Build history of the part. All positions in model axes, mm. Face numbers are marked on the shaded views. Coordinates: 2 decimals unless noted, no trailing zeros. Order: outer loops, then holes, each group sorted by start corner. A loop starts at its lowest first (then second) coordinate and runs counter-clockwise, first axis right, second up. Notation, with made-up numbers: (12.5, 55) - (56.5, 55) arc R6 ccw to (56.5, 62) - close; hole circle Ø8 at (16.5, 17.25). An arc over 180 degrees is marked (long way). Write each question's results on one line, items separated by ' | '.
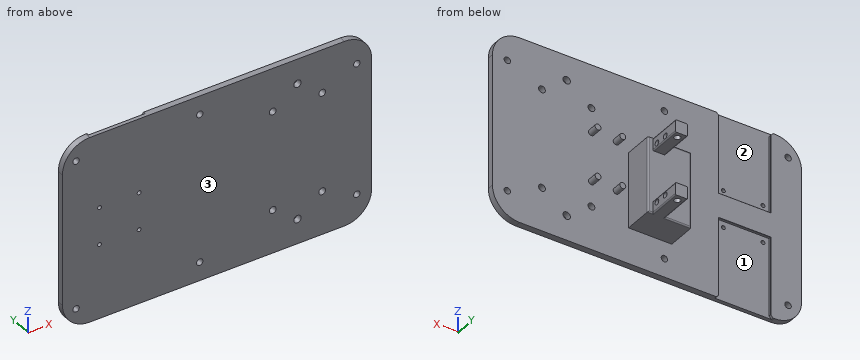
from build123d import *

# Parameters (mm, degrees)
SKETCH_1_R          = 2.6
SKETCH_1_R_2        = 3
SKETCH_1_R_3        = 2.75
EXTRUDE_1_DEPTH     = 5
SKETCH_2_W          = 42
SKETCH_2_H          = 65
CUT_EXTRUDE_1_DEPTH = 2
CHAMFER_1_SIZE      = 0.2
SKETCH_3_R          = 1.6
CUT_EXTRUDE_2_DEPTH = 3
CHAMFER_2_SIZE      = 2
SKETCH_4_R          = 2.4
EXTRUDE_2_DEPTH     = 8
SKETCH_5_W          = 35
SKETCH_5_H          = 61
EXTRUDE_3_DEPTH     = 23.5
SKETCH_7_W          = 35
SKETCH_7_H          = 10
EXTRUDE_4_DEPTH     = 30
SKETCH_8_W          = 4
SKETCH_8_H          = 10
SKETCH_8_W_2        = 21
CUT_EXTRUDE_3_DEPTH = 30
FILLET_1_R          = 1
SKETCH_9_R          = 2.2
CUT_EXTRUDE_4_DEPTH = 158.870991636
SKETCH_10_R         = 2.5
SKETCH_10_W         = 10
SKETCH_10_H         = 3
CUT_EXTRUDE_5_DEPTH = 165.764225486


with BuildPart() as part:
    # 草图1 → 凸台-拉伸1 (new body)
    with BuildSketch(Plane(origin=(0, 0, 0), x_dir=(1, 0, 0), z_dir=(0, 1, 0))):
        with BuildLine():
            Line((103, 75), (95, 75))
            Line((95, 75), (55, 75))
            Line((55, 75), (-103, 75))
            ThreePointArc((-103, 75), (-118.556349186, 68.556349186), (-125, 53))
            Line((-125, 53), (-125, -53))
            ThreePointArc((-125, -53), (-118.556349186, -68.556349186), (-103, -75))
            Line((-103, -75), (55, -75))
            Line((55, -75), (95, -75))
            Line((95, -75), (103, -75))
            ThreePointArc((103, -75), (118.556349186, -68.556349186), (125, -53))
            Line((125, -53), (125, 53))
            ThreePointArc((125, 53), (118.556349186, 68.556349186), (103, 75))
        make_face()
        with Locations(Location((-114, 60, 0), (0, 0, 270))):
            Circle(SKETCH_1_R, mode=Mode.SUBTRACT)
        with Locations(Location((-14, 60, 0), (0, 0, 270))):
            Circle(SKETCH_1_R, mode=Mode.SUBTRACT)
        with Locations(Location((113, 53, 0), (0, 0, 270))):
            Circle(SKETCH_1_R, mode=Mode.SUBTRACT)
        with Locations(Location((-114, -60, 0), (0, 0, 270))):
            Circle(SKETCH_1_R, mode=Mode.SUBTRACT)
        with Locations(Location((-14, -60, 0), (0, 0, 270))):
            Circle(SKETCH_1_R, mode=Mode.SUBTRACT)
        with Locations(Location((113, -53, 0), (0, 0, 270))):
            Circle(SKETCH_1_R, mode=Mode.SUBTRACT)
        with Locations(Location((65, -55, 0), (0, 0, 270))):
            Circle(SKETCH_1_R_2, mode=Mode.SUBTRACT)
        with Locations(Location((65, 55, 0), (0, 0, 90))):
            Circle(SKETCH_1_R_2, mode=Mode.SUBTRACT)
        with Locations(Location((45, -40, 0), (0, 0, 270))):
            Circle(SKETCH_1_R_3, mode=Mode.SUBTRACT)
        with Locations(Location((85, -40, 0), (0, 0, 270))):
            Circle(SKETCH_1_R_3, mode=Mode.SUBTRACT)
        with Locations(Location((85, 40, 0), (0, 0, 90))):
            Circle(SKETCH_1_R_3, mode=Mode.SUBTRACT)
        with Locations(Location((45, 40, 0), (0, 0, 90))):
            Circle(SKETCH_1_R_3, mode=Mode.SUBTRACT)
    extrude(amount=EXTRUDE_1_DEPTH)

    # 草图2 → 切除-拉伸1 (cut)
    with BuildSketch(Plane(origin=(0, 5, 0), x_dir=(1, 0, 0), z_dir=(0, 1, 0))):
        with Locations((-79, -42.5)):
            Rectangle(SKETCH_2_W, SKETCH_2_H)
        with Locations((-79, 42.5)):
            Rectangle(SKETCH_2_W, SKETCH_2_H)
    extrude(amount=-CUT_EXTRUDE_1_DEPTH, mode=Mode.SUBTRACT)

    # 倒角1
    chamfer_1_edges = [part.edges().sort_by_distance(p)[0] for p in [
        (-58, 5, 42.5),
        (-79, 5, 10),
        (-100, 5, -42.5),
        (-79, 5, -10),
        (-58, 5, -42.5),
        (-100, 5, 42.5),
    ]]
    chamfer(chamfer_1_edges, length=CHAMFER_1_SIZE)

    # 草图3 → 切除-拉伸2 (cut)
    with BuildSketch(Plane(origin=(0, 3, 0), x_dir=(1, 0, 0), z_dir=(0, 1, 0))):
        with Locations(Location((-95, 15, 0), (0, 0, 270))):
            Circle(SKETCH_3_R)
        with Locations(Location((-63, 15, 0), (0, 0, 270))):
            Circle(SKETCH_3_R)
        with Locations(Location((-63, -15, 0), (0, 0, 90))):
            Circle(SKETCH_3_R)
        with Locations(Location((-95, -15, 0), (0, 0, 90))):
            Circle(SKETCH_3_R)
    extrude(amount=-CUT_EXTRUDE_2_DEPTH, mode=Mode.SUBTRACT)

    # 倒角2
    chamfer_2_edges = [part.edges().sort_by_distance(p)[0] for p in [
        (-100, 3.9, -75),
        (-58, 3.9, -75),
        (-58, 3.9, 75),
        (-100, 3.9, 75),
    ]]
    chamfer(chamfer_2_edges, length=CHAMFER_2_SIZE)

    # 草图4 → 凸台-拉伸2 (add)
    with BuildSketch(Plane(origin=(0, 5, 0), x_dir=(1, 0, 0), z_dir=(0, 1, 0))):
        with Locations(Location((25, 20, 0), (0, 0, 270))):
            Circle(SKETCH_4_R)
        with Locations(Location((45, 20, 0), (0, 0, 270))):
            Circle(SKETCH_4_R)
        with Locations(Location((45, -20, 0), (0, 0, 270))):
            Circle(SKETCH_4_R)
        with Locations(Location((25, -20, 0), (0, 0, 270))):
            Circle(SKETCH_4_R)
    extrude(amount=EXTRUDE_2_DEPTH)

    # 草图5 → 凸台-拉伸3 (add)
    with BuildSketch(Plane(origin=(0, 5, 0), x_dir=(1, 0, 0), z_dir=(0, 1, 0))):
        with Locations((-2.5, 15.5)):
            Rectangle(SKETCH_5_W, SKETCH_5_H)
    extrude(amount=EXTRUDE_3_DEPTH)

    # 草图7 → 凸台-拉伸4 (add)
    with BuildSketch(Plane(origin=(0, 28.5, 0), x_dir=(1, 0, 0), z_dir=(0, 1, 0))):
        with Locations((-2.5, 41)):
            Rectangle(SKETCH_7_W, SKETCH_7_H)
        with Locations((-2.5, -10)):
            Rectangle(SKETCH_7_W, SKETCH_7_H)
    extrude(amount=EXTRUDE_4_DEPTH)

    # 草图8 → 切除-拉伸3 (cut)
    with BuildSketch(Plane(origin=(0, 58.5, 0), x_dir=(1, 0, 0), z_dir=(0, 1, 0))):
        with Locations((13, 41)):
            Rectangle(SKETCH_8_W, SKETCH_8_H)
        with Locations((-9.5, 41)):
            Rectangle(SKETCH_8_W_2, SKETCH_8_H)
        with Locations((13, -10)):
            Rectangle(SKETCH_8_W, SKETCH_8_H)
        with Locations((-9.5, -10)):
            Rectangle(SKETCH_8_W_2, SKETCH_8_H)
    extrude(amount=-CUT_EXTRUDE_3_DEPTH, mode=Mode.SUBTRACT)

    # 圆角1
    # the kernel refuses this fillet: 1 mm, written as the material it takes off along each edge
    with BuildSketch(Plane(origin=(17.5, 28.5, -46), x_dir=(0, -1, 0), z_dir=(-1, 0, 0))) as fillet_1_piece_1:
        with BuildLine():
            CenterArc((FILLET_1_R, FILLET_1_R), FILLET_1_R, 180, 90)
            Line((0, FILLET_1_R), (0, 0))
            Line((0, 0), (FILLET_1_R, 0))
        make_face()
    extrude(amount=6.5, mode=Mode.SUBTRACT)
    with BuildSketch(Plane(origin=(11, 61, -46), x_dir=(-1, 0, 0), z_dir=(0, -1, 0)), Plane(origin=(1, 61, 5), x_dir=(0, 0, 1), z_dir=(0, -1, 0)), Plane(origin=(11, 61, 5), x_dir=(-1, 0, 0), z_dir=(0, -1, 0)), Plane(origin=(11, 61, 15), x_dir=(0, 0, -1), z_dir=(0, -1, 0))) as fillet_1_piece_2:
        with BuildLine():
            CenterArc((FILLET_1_R, -FILLET_1_R), FILLET_1_R, 90, 90)
            Line((0, -FILLET_1_R), (0, 0))
            Line((0, 0), (FILLET_1_R, 0))
        make_face()
    extrude(amount=32.5, mode=Mode.SUBTRACT)
    with BuildSketch(Plane(origin=(1, 61, -46), x_dir=(1, 0, 0), z_dir=(0, -1, 0)), Plane(origin=(1, 61, -36), x_dir=(0, 0, -1), z_dir=(0, -1, 0)), Plane(origin=(11, 61, -36), x_dir=(-1, 0, 0), z_dir=(0, -1, 0)), Plane(origin=(1, 61, 15), x_dir=(0, 0, -1), z_dir=(0, -1, 0))) as fillet_1_piece_3:
        with BuildLine():
            CenterArc((FILLET_1_R, FILLET_1_R), FILLET_1_R, 180, 90)
            Line((0, FILLET_1_R), (0, 0))
            Line((0, 0), (FILLET_1_R, 0))
        make_face()
    extrude(amount=32.5, mode=Mode.SUBTRACT)
    with BuildSketch(Plane(origin=(-22.5, 28.5, -46), x_dir=(0, -1, 0), z_dir=(1, 0, 0))) as fillet_1_piece_4:
        with BuildLine():
            CenterArc((FILLET_1_R, -FILLET_1_R), FILLET_1_R, 90, 90)
            Line((0, -FILLET_1_R), (0, 0))
            Line((0, 0), (FILLET_1_R, 0))
        make_face()
    extrude(amount=23.5, mode=Mode.SUBTRACT)
    with BuildSketch(Plane(origin=(15, 28.5, -48.5), x_dir=(-1, 0, 0), z_dir=(0, 0, 1)), Plane(origin=(-20, 28.5, 17.5), x_dir=(1, 0, 0), z_dir=(0, 0, -1))) as fillet_1_piece_5:
        with BuildLine():
            CenterArc((FILLET_1_R, FILLET_1_R), FILLET_1_R, 180, 90)
            Line((0, FILLET_1_R), (0, 0))
            Line((0, 0), (FILLET_1_R, 0))
        make_face()
    extrude(amount=66, mode=Mode.SUBTRACT)
    with BuildSketch(Plane(origin=(1, 28.5, 15), x_dir=(0, 0, -1), z_dir=(-1, 0, 0))) as fillet_1_piece_6:
        with BuildLine():
            CenterArc((FILLET_1_R, FILLET_1_R), FILLET_1_R, 180, 90)
            Line((0, FILLET_1_R), (0, 0))
            Line((0, 0), (FILLET_1_R, 0))
        make_face()
    extrude(amount=23.5, mode=Mode.SUBTRACT)
    with BuildSketch(Plane(origin=(17.5, 28.5, -46), x_dir=(0, -1, 0), z_dir=(-1, 0, 0))) as fillet_1_piece_7a_section:
        with BuildLine():
            CenterArc((FILLET_1_R, FILLET_1_R), FILLET_1_R, 180, 90)
            Line((0, FILLET_1_R), (0, 0))
            Line((0, 0), (FILLET_1_R, 0))
        make_face()
    fillet_1_piece_7a = extrude(amount=9, mode=Mode.PRIVATE)
    fillet_1_piece_7a = split(fillet_1_piece_7a, bisect_by=Plane(origin=(11, 28.273604886, -45.773604886), z_dir=(-1, 0, 0)), keep=Keep.TOP, mode=Mode.PRIVATE)
    with BuildSketch(Plane(origin=(11, 61, -46), x_dir=(-1, 0, 0), z_dir=(0, -1, 0))) as fillet_1_piece_7b_section:
        with BuildLine():
            CenterArc((FILLET_1_R, -FILLET_1_R), FILLET_1_R, 90, 90)
            Line((0, -FILLET_1_R), (0, 0))
            Line((0, 0), (FILLET_1_R, 0))
        make_face()
    fillet_1_piece_7b = extrude(amount=35, mode=Mode.PRIVATE)
    fillet_1_piece_7b = split(fillet_1_piece_7b, bisect_by=Plane(origin=(10.773604886, 28.5, -45.773604886), z_dir=(0, -1, 0)), keep=Keep.TOP, mode=Mode.PRIVATE)
    fillet_1_piece_7 = fillet_1_piece_7a & fillet_1_piece_7b
    add(fillet_1_piece_7, mode=Mode.SUBTRACT)
    with BuildSketch(Plane(origin=(1, 61, -46), x_dir=(1, 0, 0), z_dir=(0, -1, 0))) as fillet_1_piece_8a_section:
        with BuildLine():
            CenterArc((FILLET_1_R, FILLET_1_R), FILLET_1_R, 180, 90)
            Line((0, FILLET_1_R), (0, 0))
            Line((0, 0), (FILLET_1_R, 0))
        make_face()
    fillet_1_piece_8a = extrude(amount=35, mode=Mode.PRIVATE)
    fillet_1_piece_8a = split(fillet_1_piece_8a, bisect_by=Plane(origin=(1.226395114, 28.5, -45.773604886), z_dir=(0, -1, 0)), keep=Keep.TOP, mode=Mode.PRIVATE)
    with BuildSketch(Plane(origin=(-22.5, 28.5, -46), x_dir=(0, -1, 0), z_dir=(1, 0, 0))) as fillet_1_piece_8b_section:
        with BuildLine():
            CenterArc((FILLET_1_R, -FILLET_1_R), FILLET_1_R, 90, 90)
            Line((0, -FILLET_1_R), (0, 0))
            Line((0, 0), (FILLET_1_R, 0))
        make_face()
    fillet_1_piece_8b = extrude(amount=26, mode=Mode.PRIVATE)
    fillet_1_piece_8b = split(fillet_1_piece_8b, bisect_by=Plane(origin=(1, 28.273604886, -45.773604886), z_dir=(1, 0, 0)), keep=Keep.TOP, mode=Mode.PRIVATE)
    fillet_1_piece_8 = fillet_1_piece_8a & fillet_1_piece_8b
    add(fillet_1_piece_8, mode=Mode.SUBTRACT)
    with BuildSketch(Plane(origin=(3.5, 28.5, 15), x_dir=(0, 0, -1), z_dir=(-1, 0, 0))) as fillet_1_piece_9a_section:
        with BuildLine():
            CenterArc((FILLET_1_R, FILLET_1_R), FILLET_1_R, 180, 90)
            Line((0, FILLET_1_R), (0, 0))
            Line((0, 0), (FILLET_1_R, 0))
        make_face()
    fillet_1_piece_9a = extrude(amount=26, mode=Mode.PRIVATE)
    fillet_1_piece_9a = split(fillet_1_piece_9a, bisect_by=Plane(origin=(1, 28.273604886, 14.773604886), z_dir=(1, 0, 0)), keep=Keep.TOP, mode=Mode.PRIVATE)
    with BuildSketch(Plane(origin=(1, 61, 15), x_dir=(0, 0, -1), z_dir=(0, -1, 0))) as fillet_1_piece_9b_section:
        with BuildLine():
            CenterArc((FILLET_1_R, FILLET_1_R), FILLET_1_R, 180, 90)
            Line((0, FILLET_1_R), (0, 0))
            Line((0, 0), (FILLET_1_R, 0))
        make_face()
    fillet_1_piece_9b = extrude(amount=35, mode=Mode.PRIVATE)
    fillet_1_piece_9b = split(fillet_1_piece_9b, bisect_by=Plane(origin=(1.226395114, 28.5, 14.773604886), z_dir=(0, -1, 0)), keep=Keep.TOP, mode=Mode.PRIVATE)
    fillet_1_piece_9 = fillet_1_piece_9a & fillet_1_piece_9b
    add(fillet_1_piece_9, mode=Mode.SUBTRACT)

    # 草图9 → 切除-拉伸4 (cut, through all)
    with BuildSketch(Plane.ZY.offset(-1)):
        with Locations((-39.5, 43.3)):
            Circle(SKETCH_9_R)
        with Locations((-39.5, 33.3)):
            Circle(SKETCH_9_R)
        with Locations((8.5, 43.3)):
            Circle(SKETCH_9_R)
        with Locations((8.5, 33.3)):
            Circle(SKETCH_9_R)
    extrude(amount=-CUT_EXTRUDE_4_DEPTH, mode=Mode.SUBTRACT)

    # 草图10 → 切除-拉伸5 (cut, through all)
    with BuildSketch(Plane.XY.offset(15)):
        with Locations((6, 50.5)):
            Circle(SKETCH_10_R)
        with Locations((6, 57)):
            Rectangle(SKETCH_10_W, SKETCH_10_H)
    extrude(amount=-CUT_EXTRUDE_5_DEPTH, mode=Mode.SUBTRACT)


solid = part.part
1. Band-saw the part on B-B on z = 40. Give the cut face in (x, y).
Solved:
outline: (-125, 0) - (42.25, 0) - (42.25, 5) - (-57.8, 5) - (-58, 4.8) - (-58, 3) - (-100, 3) - (-100, 4.8) - (-100.2, 5) - (-125, 5) - close; (47.75, 0) - (82.25, 0) - (82.25, 5) - (47.75, 5) - close; (87.75, 0) - (125, 0) - (125, 5) - (87.75, 5) - close
2. Two-plate mould, pull along X, no slides. Class the marked faces 1, 2 and 3: +X half, -X half, draft (parallel to the pull), parting line (faces both ways), or undercut.
Solved:
face 1: undercut | face 2: undercut | face 3: draft
3. Band-saw the part on C-C on z = -20. Give the cut face in (x, y), then the cut area to 3 significant figures.
Solved:
outline: (-125, 0) - (125, 0) - (125, 5) - (47.4, 5) - (47.4, 13) - (42.6, 13) - (42.6, 5) - (27.4, 5) - (27.4, 13) - (22.6, 13) - (22.6, 5) - (15, 5) - (15, 27.5) arc R1 ccw to (14, 28.5) - (-19, 28.5) arc R1 ccw to (-20, 27.5) - (-20, 5) - (-57.8, 5) - (-58, 4.8) - (-58, 3) - (-100, 3) - (-100, 4.8) - (-100.2, 5) - (-125, 5) - close | area: 2,060 mm2
4. Band-saw the part on D-D on x = -76.5. Give the cut face in (y, z), then the cut area to 3 significant figures.
Solved:
outline: (0, -75) - (3, -75) - (3, -10) - (4.8, -10) - (5, -9.8) - (5, 9.8) - (4.8, 10) - (3, 10) - (3, 75) - (0, 75) - close | area: 490 mm2
5. Probe line 1 (X direction, y = 0.6, z = -15); line 2 (Z direction, x = -95, y = 1); line 3 (X direction, y = 2, z = 60). List the from-to ranges inside material, lowest first.
Solved:
line 1: x = -125 to -96.6, -93.4 to -64.6, -61.4 to 125 | line 2: z = -75 to -16.6, -13.4 to 13.4, 16.6 to 75 | line 3: x = -123.86 to -116.6, -111.4 to -16.6, -11.4 to 123.86
6. Drop flat-ended pins along their axis: pin 1 Ø6.5 at (x, y) = (7.5, 45.5) entering from -Z; pin 2 Ø9 at (y, z) = (44, -40) entering from +X; pin 3 Ø7 at (x, z) = (113, -53) entering from +Y. Give the stop position or say it passes through.
Solved:
pin 1: stops at z = -46 | pin 2: stops at x = 11 | pin 3: stops at y = 5
7. Band-saw the part on A-A on x = 65. Give the cut face in (y, z).
Solved:
outline: (0, -75) - (5, -75) - (5, -58) - (0, -58) - close; (0, -52) - (5, -52) - (5, 52) - (0, 52) - close; (0, 58) - (5, 58) - (5, 75) - (0, 75) - close
